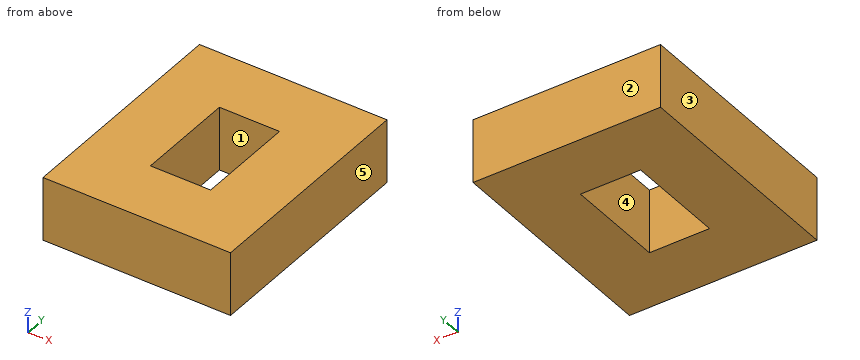
Autodesk Inventor part; units mm, degrees
ref_plane "YZ Plane" through (0, 0, 0) normal (1, 0, 0) x (0, 1, 0)
ref_plane "XZ Plane" through (0, 0, 0) normal (0, 1, 0) x (-1, 0, 0)
ref_plane "XY Plane" through (0, 0, 0) normal (0, 0, 1) x (1, 0, 0)
sketch "Sketch1" plane through (0, 0, 0) normal (0, 0, 1) x (1, 0, 0)
  line L0 (-1.5, 2.5) -> (1.5, 2.5)
  line L1 (1.5, 2.5) -> (1.5, -2.5)
  line L2 (1.5, -2.5) -> (-1.5, -2.5)
  line L3 (-1.5, -2.5) -> (-1.5, 2.5)
  line L4 (-1.5, 2.5) -> (1.5, -2.5) construction
  line L5 (1.5, 2.5) -> (-1.5, -2.5) construction
  line L6 (4.675, 5.675) -> (-4.675, 5.675)
  line L7 (-4.675, 5.675) -> (-4.675, -5.675)
  line L8 (-4.675, -5.675) -> (4.675, -5.675)
  line L9 (4.675, -5.675) -> (4.675, 5.675)
  point P0 (0, 0)
  dimension "d0" = 3
  dimension "d1" = 5
  dimension "d2" = 3.175
extrude "Extrusion1" add sketch "Sketch1" along normal mid plane 3.175
properties part number "Motor Fitting Test"
Can you work these out from the model? Positions are in its coordinate system, mm. Face numbers are marked on the shaded views. A direction names the side the tool comes from. Coordinates: 2 decimals unless noted, no trailing zeros. Order: outer loops, then holes, each group sorted by start corner. A loop starts at its lowest first (then second) coordinate and runs counter-clockwise, first axis right, second up. Notation, with made-up numbers: (11, -8.5) - (70, -8.5) arc R24 cw to (70, 3.5) - close; hole circle Ø10 at (42.25, 11.5). An arc over 180 degrees is marked (long way). Answer in a Markdown table with one row per item.
1. For the marked faces 4 and 5, which set-ups out of +Z, -Z, +X, -X, +Y, -Y let a thin tool reach every point of the face, with its end or its side?
Reply:
| item | result |
|---|---|
| face 4 | +Z, -Z |
| face 5 | +Z, -Z, +X, +Y, -Y |
2. Suppose I cut it at A-A (y = -1.25). Please give me the cut outline in (x, z) (1 decimal), and give its area (3 significant figures).
Reply:
| item | result |
|---|---|
| outline | (-4.7, -1.6) - (-1.5, -1.6) - (-1.5, 1.6) - (-4.7, 1.6) - close; (1.5, -1.6) - (4.7, -1.6) - (4.7, 1.6) - (1.5, 1.6) - close |
| area | 20.2 mm^2 |
3. Suppose I cut it at B-B (x = 0.5). Please give me the cut outline in (y, z) (1 decimal), and give its area (3 significant figures).
Reply:
| item | result |
|---|---|
| outline | (-5.7, -1.6) - (-2.5, -1.6) - (-2.5, 1.6) - (-5.7, 1.6) - close; (2.5, -1.6) - (5.7, -1.6) - (5.7, 1.6) - (2.5, 1.6) - close |
| area | 20.2 mm^2 |
4. If we mould it in two halves opening along Y, with no side actions, what happens to the marked faces 1, 2 and 3? For each: pulls with the +Y half, pulls with the -Y half, needs draft (parallel to the pull), parting line crosses it, or undercut.
Reply:
| item | result |
|---|---|
| face 1 | undercut |
| face 2 | pulls with the +Y half |
| face 3 | needs draft |
5. Suppose I cut it at C-C (z = 0). Please give me the cut outline in (x, y) (3 decimals).
Reply:
| item | result |
|---|---|
| outline | (-4.675, -5.675) - (4.675, -5.675) - (4.675, 5.675) - (-4.675, 5.675) - close; hole (-1.5, -2.5) - (1.5, -2.5) - (1.5, 2.5) - (-1.5, 2.5) - close |
6. If I drill on line 1 along X through (y, z) = (-0.5, 1.15) (3 decimals); line 2 along Y through (x, z) = (0.5, -0.2) (3 decimals), over which ranges is the centre line in solid material (lowest first)?
Reply:
| item | result |
|---|---|
| line 1 | x = -4.675 to -1.5, 1.5 to 4.675 |
| line 2 | y = -5.675 to -2.5, 2.5 to 5.675 |
